from build123d import *

# Parameters (mm, degrees)
BOSS_EXTRUDE1_DEPTH = 42
BOSS_EXTRUDE2_DEPTH = 5


with BuildPart() as part:
    # Sketch1 → Boss-Extrude1 (new body)
    with BuildSketch(Plane.XY):
        with BuildLine():
            Line((75, 0), (70, 0))
            ThreePointArc((70, 0), (0, -70), (-70, 0))
            Line((-70, 0), (-75, 0))
            ThreePointArc((-75, 0), (0, -75), (75, 0))
        make_face()
    extrude(amount=BOSS_EXTRUDE1_DEPTH)

    # Sketch2 → Boss-Extrude2 (add)
    with BuildSketch(Plane.XY.offset(42)):
        with BuildLine():
            Line((75, 0), (70, 0))
            ThreePointArc((70, 0), (0, -70), (-70, 0))
            Line((-70, 0), (-75, 0))
            ThreePointArc((-75, 0), (0, -75), (75, 0))
        make_face()
        with BuildLine():
            Line((-40, 0), (-70, 0))
            ThreePointArc((-70, 0), (0, -70), (70, 0))
            Line((70, 0), (40, 0))
            ThreePointArc((40, 0), (0, -40), (-40, 0))
        make_face()
    extrude(amount=BOSS_EXTRUDE2_DEPTH)


solid = part.part
Geometry check sheet. Reference: the model listing, model coordinates, mm. A direction names the side the tool comes from. Give positions to 0.01 mm unless a question says otherwise; leave off trailing zeros. Order: outer loops, then holes, each group sorted by start corner. A loop starts at its lowest first (then second) coordinate and runs counter-clockwise, first axis right, second up. Notation, with made-up numbers: M -24.5,75.25 L 20.5,75.25 A19 ccw 20.5,98.25 Z; hole C 9.25,4 d7. An arc over 180 degrees is marked long. Use a Markdown table: item, result.
Item 1: Depth check by flat-ended pin: P1, Ø1.5, axis at y = -51, z = 35, coming from the -X side; P2, Ø4, axis at y = -37.5, z = 15.5, coming from the -X side; P3, Ø10, axis at x = -7.5, y = -40.5, coming from the -Z side. Enter the tip coordinate at first touch or a pass-through.
Answers follow:
| item | result |
|---|---|
| P1 | stops at x = -55.68 |
| P2 | stops at x = -66.07 |
| P3 | stops at z = 42 |
Item 2: Draft check along X on faces 1 (the cylindrical face through (1.539, -69.983, 20.706)), 2 (the flat face through (0, -71, 0)), 3 (the cylindrical face through (-1.65, -74.98, 23.17)). Enter one of: +X half, -X half, draft (parallel to the pull), parting line (faces both ways), or undercut.
Answers follow:
| item | result |
|---|---|
| face 1 | undercut |
| face 2 | draft |
| face 3 | parting line |
Item 3: Section check B-B (x = 0). Record the cut outline in (y, z).
Answers follow:
| item | result |
|---|---|
| outline | M -75,0 L -70,0 L -70,42 L -40,42 L -40,47 L -75,47 Z |
Item 4: Section check A-A (y = -9.5). Record the cut outline in (x, z), and give its area (3 significant figures).
Answers follow:
| item | result |
|---|---|
| outline | M -74.4,0 L -69.35,0 L -69.35,42 L -38.86,42 L -38.86,47 L -74.4,47 Z; M 38.86,42 L 69.35,42 L 69.35,0 L 74.4,0 L 74.4,47 L 38.86,47 Z |
| area | 779 mm2 |
Item 5: Section check C-C (z = 32.5). Record the cut outline in (x, y), and give its area (3 significant figures).
Answers follow:
| item | result |
|---|---|
| outline | M -75,0 A75 ccw 75,0 L 70,0 A70 cw -70,0 Z |
| area | 1,140 mm2 |
Item 6: Material ranges on line 1 along Z through (x, y) = (42.5, -37.5); line 2 along X through (y, z) = (-32, 23); line 3 along X through (y, z) = (-44, 6.5), recorded low to high.
Answers follow:
| item | result |
|---|---|
| line 1 | z = 42 to 47 |
| line 2 | x = -67.83 to -62.26, 62.26 to 67.83 |
| line 3 | x = -60.74 to -54.44, 54.44 to 60.74 |
Item 7: Tool access check on faces 4 (the flat face through (-1, -42, 42)), 5 (the cylindrical face through (0.88, -39.99, 44.46)). Record the directions out of +Z, -Z, +X, -X, +Y, -Y that give a thin tool (end or side, any length) a straight path to the whole face; none if there is none.
Answers follow:
| item | result |
|---|---|
| face 4 | -Z, +Y |
| face 5 | +Z, -Z, +Y |
Item 8: Section check D-D (y = -44.5). Record the cut outline in (x, z).
Answers follow:
| item | result |
|---|---|
| outline | M -60.37,0 L -54.03,0 L -54.03,42 L 54.03,42 L 54.03,0 L 60.37,0 L 60.37,47 L -60.37,47 Z |
